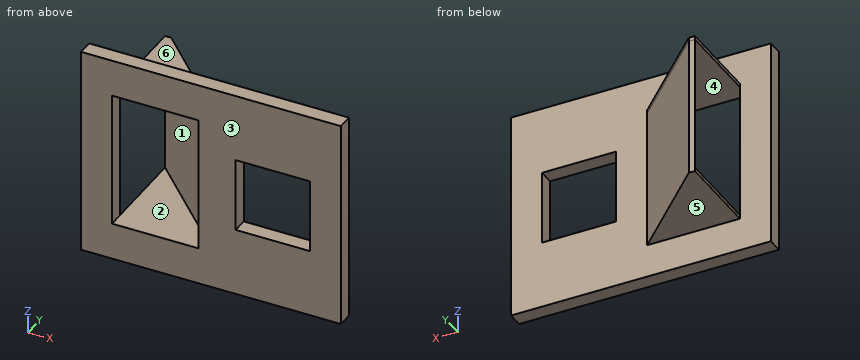
from build123d import *

# Parameters (mm, degrees)
SKETCH_1_W          = 210
SKETCH_1_H          = 170
EXTRUDE_1_DEPTH     = 12.5
SKETCH_2_W          = 60
SKETCH_2_H          = 60
CUT_EXTRUDE_1_DEPTH = 15
SKETCH_3_W          = 70
SKETCH_3_H          = 110
CUT_EXTRUDE_4_DEPTH = 20
EXTRUDE_4_DEPTH     = 5
EXTRUDE_6_DEPTH     = 3
EXTRUDE_7_DEPTH     = 3
EXTRUDE_8_DEPTH     = 3
EXTRUDE_9_DEPTH     = 3


with BuildPart() as part:
    # Эскиз1 → Бобышка-Вытянуть1 (new body)
    with BuildSketch(Plane(origin=(0, 0, 0), x_dir=(1, 0, 0), z_dir=(0, 1, 0))):
        Rectangle(SKETCH_1_W, SKETCH_1_H)
    extrude(amount=EXTRUDE_1_DEPTH)

    # Эскиз2 → Вырез-Вытянуть1 (cut)
    with BuildSketch(Plane(origin=(0, 12.5, 0), x_dir=(1, 0, 0), z_dir=(0, 1, 0))):
        with Locations((50, 0)):
            Rectangle(SKETCH_2_W, SKETCH_2_H)
    extrude(amount=-CUT_EXTRUDE_1_DEPTH, mode=Mode.SUBTRACT)

    # Эскиз3 → Вырез-Вытянуть4 (cut)
    with BuildSketch(Plane(origin=(0, 0, 0), x_dir=(1, 0, 0), z_dir=(0, 1, 0))):
        with Locations((-45, 0)):
            Rectangle(SKETCH_3_W, SKETCH_3_H)
    extrude(amount=CUT_EXTRUDE_4_DEPTH, mode=Mode.SUBTRACT)

    # Sketch 1 2 → Бобышка-Вытянуть4 (add, along a direction that is not the sketch's normal)
    with BuildSketch(Plane(origin=(-10, 12.5, -55), x_dir=(-0.47301616487964127, 0.4730161648796364, 0.7433111162394362), z_dir=(0.7071067811865439, 0.7071067811865512, 0))):
        Polygon((0, 0), (81.764222786, 73.584046315), (147.986485869, 0), (66.222263083, -73.584046315), align=None)
    extrude(amount=EXTRUDE_4_DEPTH, dir=(1, 0, 0))

    # Sketch 3 2 → Бобышка-Вытянуть6 (add)
    with BuildSketch(Plane(origin=(-7.5, 12.5, -55), x_dir=(-0.7194014606174125, 0.6945945136995638, 0), z_dir=(0, 0, 1))):
        Polygon((0, 0), (52.156605895, 50.358102243), (100.778221854, 0), align=None)
    extrude(amount=-EXTRUDE_6_DEPTH)

    # Sketch 4 → Бобышка-Вытянуть7 (add)
    with BuildSketch(Plane(origin=(-7.5, 12.5, 55), x_dir=(-0.7194014606174126, 0.6945945136995636, 0), z_dir=(0, 0, 1))):
        Polygon((0, 0), (100.778221854, 0), (52.156605895, 50.358102243), align=None)
    extrude(amount=EXTRUDE_7_DEPTH)

    # Эскиз7 → Бобышка-Вытянуть8 (add)
    with BuildSketch(Plane(origin=(0, 0, -55), x_dir=(-1, 0, 0), z_dir=(0, 0, -1))):
        Polygon((5, 12.5), (7.5, 12.5), (80, 82.5), (75, 82.5), align=None)
    extrude(amount=EXTRUDE_8_DEPTH)

    # Sketch 5 → Бобышка-Вытянуть9 (add)
    with BuildSketch(Plane(origin=(-5, 12.5, 55), x_dir=(-0.7310552682428726, 0.6823182503600075, 0), z_dir=(0, 0, -1))):
        Polygon((0, 0), (1.827638171, -1.705795626), (102.591422643, 0), (98.936146302, 3.411591252), align=None)
    extrude(amount=-EXTRUDE_9_DEPTH)


solid = part.part
Part model, mm, in its own coordinate system. Face numbers are marked on the shaded views. A direction names the side the tool comes from. Round coordinates to 2 decimals unless told otherwise and drop trailing zeros. Write each loop counter-clockwise with the first axis right and the second up, starting at its lowest first coordinate (ties: lowest second). Pieces come first, ordered by that corner, then holes. Notation, with made-up numbers: M 49.25,-6.5 L 89.25,-6.5 A14 cw 89.25,-0.5 Z; hole C 87.25,55 d10. An arc over 180 degrees is marked long. Return JSON: item names as keys, results as strings. Group by question number.
(1) Saw through at A-A on y = 9. Write the cut outline in (x, z), then the cut area to 3 significant figures.
(2) Pin check, flat tips, straight feed: pin 1 Ø1.5 at (y, z) = (14, -44) entering from -X; pin 2 Ø12 at (x, z) = (-36.5, -63) entering from +Y; pin 3 Ø2.5 at (y, z) = (30, 56) entering from -X. Stop position of each tip, or through.
(3) Saw through at C-C on x = 60. Write the cut outline in (y, z).
(4) Which spindle directions (+Z, -Z, +X, -X, +Y, -Y) get a long thin tool onto all of the face, cutting with end or side? Do the marked faces 1 and 2. Say none if no direction does.
(5) Saw through at D-D on x = -53. Write the cut outline in (y, z).
(6) Two-plate mould, pull along Z, no slides. Class the marked faces 3, 4, 5 and 6: +Z half, -Z half, draft (parallel to the pull), parting line (faces both ways), or undercut.
(7) Drill centre lines: probe 1 along X at (y, z) = (12, 1); probe 2 along Z at (x, y) = (-60, 23.5); probe 3 along X at (y, z) = (4, -47). Where is each one in solid material? Low to high.
(8) Saw through at B-B on z = -41. Write the cut outline in (x, y).
Returned:
{
 "1": {"outline": "M -105,-85 L 105,-85 L 105,85 L -105,85 Z; hole M -80,-55 L -10,-55 L -10,55 L -80,55 Z; hole M 20,-30 L 80,-30 L 80,30 L 20,30 Z", "area": "24,400 mm²"},
 "2": {"pin 1": "x = -12.25", "pin 2": "y = 47.32", "pin 3": "x = -80"},
 "3": {"outline": "M 0,-85 L 12.5,-85 L 12.5,-30 L 0,-30 Z; M 0,30 L 12.5,30 L 12.5,85 L 0,85 Z"},
 "4": {"face 1": "-X, -Y", "face 2": "-Y"},
 "5": {"outline": "M 0,-85 L 12.5,-85 L 12.5,-58 L 60.5,-58 L 60.5,58 L 12.5,58 L 12.5,85 L 0,85 L 0,55 L 55.5,55 L 55.5,-55 L 0,-55 Z"},
 "6": {"face 3": "draft", "face 4": "undercut", "face 5": "-Z half", "face 6": "+Z half"},
 "7": {"probe 1": "-105 to -80, -10 to 20, 80 to 105", "probe 2": "-58 to -55, 55 to 58", "probe 3": "-105 to -80, -10 to 105"},
 "8": {"outline": "M -105,0 L -80,0 L -80,12.5 L -105,12.5 Z; M -80,82.5 L -10,12.5 L -10,0 L 105,0 L 105,12.5 L -5,12.5 L -75,82.5 Z"}
}
